Read the model definition and answer for the solid it produces. Units are mm, in the model's axes. A direction names the side the tool comes from. Coordinates: 2 decimals unless noted, no trailing zeros. Order: outer loops, then holes, each group sorted by start corner. A loop starts at its lowest first (then second) coordinate and runs counter-clockwise, first axis right, second up. Notation, with made-up numbers: (-6.75, 33.5) -> (22.25, 33.5) arc R26 cw to (22.25, 57.5) -> close; hole circle Ø2 at (31.25, -40). An arc over 180 degrees is marked (long way). Answer in a Markdown table with one row per item.
from build123d import *

# Parameters (mm, degrees)
SKETCH1_W           = 276
SKETCH1_H           = 456
BOSS_EXTRUDE1_DEPTH = 25
SKETCH2_W           = 28
SKETCH2_H           = 28
SKETCH2_H_2         = 192
CUT_EXTRUDE1_DEPTH  = 25


with BuildPart() as part:
    # Sketch1 → Boss-Extrude1 (new body)
    with BuildSketch(Plane(origin=(0, 0, 0), x_dir=(0, 0, -1), z_dir=(1, 0, 0))):
        with Locations((-123.692307692, 18.538461538)):
            Rectangle(SKETCH1_W, SKETCH1_H)
    extrude(amount=BOSS_EXTRUDE1_DEPTH)

    # Sketch2 → Cut-Extrude1 (cut)
    with BuildSketch(Plane(origin=(0, 0, 0), x_dir=(0, 0, -1), z_dir=(1, 0, 0))):
        with Locations((0.307692308, -195.461538462)):
            Rectangle(SKETCH2_W, SKETCH2_H)
        with Locations((-247.692307692, -195.461538462)):
            Rectangle(SKETCH2_W, SKETCH2_H)
        with Locations((0.307692308, 232.538461538)):
            Rectangle(SKETCH2_W, SKETCH2_H)
        with Locations((-247.692307692, 232.538461538)):
            Rectangle(SKETCH2_W, SKETCH2_H)
        with Locations((0.307692308, 18.538461538)):
            Rectangle(SKETCH2_W, SKETCH2_H_2)
        with Locations((-247.692307692, 18.538461538)):
            Rectangle(SKETCH2_W, SKETCH2_H_2)
    extrude(amount=CUT_EXTRUDE1_DEPTH, mode=Mode.SUBTRACT)


solid = part.part
Q1. Consider line 1 (Y direction, x = 23, z = 7); line 2 (Z direction, x = 14, y = 46). Determine where each line is inside the solid, lowest interval first.
Outcome:
| item | result |
|---|---|
| line 1 | -181.46 to -77.46, 114.54 to 218.54 |
| line 2 | 13.69 to 233.69 |
Q2. The part is cut by section A-A (z = 241). Write down the section's boundary in (x, y), then the cut area to 3 significant figures.
Outcome:
| item | result |
|---|---|
| outline | (0, -181.46) -> (25, -181.46) -> (25, -77.46) -> (0, -77.46) -> close; (0, 114.54) -> (25, 114.54) -> (25, 218.54) -> (0, 218.54) -> close |
| area | 5,200 mm² |
Q3. The part is cut by section B-B (x = 15). Write down the section's boundary in (y, z), then the cut area to 3 significant figures.
Outcome:
| item | result |
|---|---|
| outline | (-209.46, 13.69) -> (-181.46, 13.69) -> (-181.46, -14.31) -> (-77.46, -14.31) -> (-77.46, 13.69) -> (114.54, 13.69) -> (114.54, -14.31) -> (218.54, -14.31) -> (218.54, 13.69) -> (246.54, 13.69) -> (246.54, 233.69) -> (218.54, 233.69) -> (218.54, 261.69) -> (114.54, 261.69) -> (114.54, 233.69) -> (-77.46, 233.69) -> (-77.46, 261.69) -> (-181.46, 261.69) -> (-181.46, 233.69) -> (-209.46, 233.69) -> close |
| area | 112,000 mm² |
Q4. For faces 1 (the face through (12, -77.462, 248)), 2 (the face through (12, 232, 13.692)), 3 (the face through (12, -77.462, 0)), 4 (the face through (12, 232, 233.692)), determine the directions among +Z, -Z, +X, -X, +Y, -Y from which every point of the face is accessible in a straight line to the end or side of a thin tool.
Outcome:
| item | result |
|---|---|
| face 1 | +Z, +X, -X |
| face 2 | -Z, +X, -X, +Y |
| face 3 | -Z, +X, -X |
| face 4 | +Z, +X, -X, +Y |
Q5. The part is cut by section C-C (y = -6). Write down the section's boundary in (x, z), then the cut area to 3 significant figures.
Outcome:
| item | result |
|---|---|
| outline | (0, 13.69) -> (25, 13.69) -> (25, 233.69) -> (0, 233.69) -> close |
| area | 5,500 mm² |
Q6. Given pin 1 (5 mm diameter, centred on y = -138.5, z = 211, fed in from -X); pin 2 (12.5 mm diameter, centred on x = 15.5, z = 254, fed in from -Y); pin 3 (7.5 mm diameter, centred on x = 14, z = 4, fed in from +Y); pin 4 (4 mm diameter, centred on x = 6.5, y = -51, fed in from +Z), each flat-ended and moving along its own axis, determine where each tip first touches the part or whether it passes through.
Outcome:
| item | result |
|---|---|
| pin 1 | x = 0 |
| pin 2 | y = -181.46 |
| pin 3 | y = 218.54 |
| pin 4 | z = 233.69 |
